Geometry check sheet. Reference: the model listing, model coordinates, mm. A direction names the side the tool comes from. Round coordinates to 2 decimals unless told otherwise and drop trailing zeros. Write each loop counter-clockwise with the first axis right and the second up, starting at its lowest first coordinate (ties: lowest second). Pieces come first, ordered by that corner, then holes. Notation, with made-up numbers: M 3,74.5 L 40,74.5 A22 cw 40,96.5 Z; hole C -3.75,-22 d1. An arc over 180 degrees is marked long. One line per item, written item: value. Start each with the question number.
1. Depth check by flat-ended pin: P1, Ø8.5, axis at x = 0.5, z = 1, coming from the -Y side; P2, Ø3, axis at x = 0, z = 0, coming from the +Y side; P3, Ø3.5, axis at x = -14, y = 20, coming from the +Z side; P4, Ø1, axis at x = -11.5, z = 4.5, coming from the -Y side. Enter the tip coordinate at first touch or a pass-through.
2. Section check B-B (x = 0). Record the boundary of the cut face in (y, z).
3. Section check D-D (z = -19). Record the boundary of the cut face in (x, y).
4. Scan lines: probe 1 along X at (y, z) = (11.5, 0); probe 2 along Y at (x, z) = (-14, 3); probe 3 along Y at (x, z) = (-5, -3.5). Record each from-to range of solid material in increasing order. Write a range as [from, to].
5. Access from +Z, -Z, +X, -X, +Y, -Y to the whole of each face (thin tool, end or side, straight path). Record for faces 1 (the cylindrical face through (19.16, 65.06, -25.94)), 2 (the cylindrical face through (2.54, 9.92, 8.06)), 3 (the flat face through (-13, 22, 9.5)).
from build123d import *

# Parameters (mm, degrees)
SKETCH_1_R           = 5.95
EXTRUDE_1_DEPTH      = 4.5
SKETCH_4_R           = 8.45
EXTRUDE_4_DEPTH      = 17.75
EXTRUDE_6_DEPTH      = 5.75
EXTRUDE_6_DEPTH_BACK = 5.75
SKETCH_12_R          = 9.5
EXTRUDE_10_DEPTH     = 1
SKETCH_7_R           = 2.3
CUT_EXTRUDE_1_DEPTH  = 57.22806055
SKETCH_8_R           = 6.5
CUT_EXTRUDE_2_DEPTH  = 6
SKETCH_9_R           = 9.5
EXTRUDE_7_DEPTH      = 36
SKETCH_10_R          = 8.45
EXTRUDE_8_DEPTH      = 40
EXTRUDE_START        = 1
SKETCH_13_R          = 9.5
SKETCH_13_R_2        = 2.3
EXTRUDE_11_DEPTH     = 1
SKETCH_14_R          = 3.25
CUT_EXTRUDE_3_DEPTH  = 8
CUT_EXTRUDE_START    = -18
CUT_EXTRUDE_4_DEPTH  = 18
CUT_EXTRUDE_START_2  = 11
SKETCH_16_R          = 14.956390748
SKETCH_16_R_2        = 7.5
CUT_EXTRUDE_5_DEPTH  = 22
FILLET_2_R           = 5
SKETCH_18_R          = 7.5
EXTRUDE_12_DEPTH     = 11.5


with BuildPart() as part:
    # Эскиз1 → Бобышка-Вытянуть1 (new body)
    with BuildSketch(Plane(origin=(0, 0, 0), x_dir=(1, 0, 0), z_dir=(0, 1, 0))):
        with Locations(Location((0, 0, 0), (0, 0, 270))):
            Circle(SKETCH_1_R)
    extrude(amount=EXTRUDE_1_DEPTH)

    # Эскиз4 → Бобышка-Вытянуть4 (add)
    with BuildSketch(Plane(origin=(0, 4.5, 0), x_dir=(1, 0, 0), z_dir=(0, 1, 0))):
        with Locations(Location((0, 0, 0), (0, 0, 270))):
            Circle(SKETCH_4_R)
    extrude(amount=EXTRUDE_4_DEPTH)

    # Эскиз6 → Бобышка-Вытянуть6 (add, two sides: drawn at the far end of the back side and taken through both)
    with BuildSketch(Plane(origin=(0, 22.25, 0), x_dir=(1, 0, 0), z_dir=(0, 1, 0)).offset(-EXTRUDE_6_DEPTH_BACK)):
        with BuildLine():
            Line((-7.002075382, 9.5), (-30, 9.5))
            Line((-30, 9.5), (-30, -9.5))
            Line((-30, -9.5), (0, -9.5))
            Line((0, -9.5), (0.833655922, -9.5))
            ThreePointArc((0.833655922, -9.5), (3.331132848, -9.18310947), (5.670324417, -8.252521801))
            ThreePointArc((5.670324417, -8.252521801), (13.556905273, -2.05094269), (19.066851837, 6.333461279))
            Line((19.066851837, 6.333461279), (28.114764095, 31.1923959))
            Line((28.114764095, 31.1923959), (10.2606043, 37.690778624))
            Line((10.2606043, 37.690778624), (2.394850826, 16.079798567))
            ThreePointArc((2.394850826, 16.079798567), (-1.266311019, 11.308479557), (-7.002075382, 9.5))
        make_face()
    extrude(amount=EXTRUDE_6_DEPTH + EXTRUDE_6_DEPTH_BACK)

    # Эскиз12 → Бобышка-Вытянуть10 (add)
    with BuildSketch(Plane(origin=(0, 28, 0), x_dir=(1, 0, 0), z_dir=(0, 1, 0))):
        with Locations(Location((15.938492836, 25.514507365, 0), (0, 0, 70))):
            Circle(SKETCH_12_R)
    extrude(amount=EXTRUDE_10_DEPTH)

    # Эскиз7 → Вырез-Вытянуть1 (cut, through all)
    with BuildSketch(Plane.XZ):
        with Locations(Location((0, 0, 0), (0, 0, 270))):
            Circle(SKETCH_7_R)
    extrude(amount=-CUT_EXTRUDE_1_DEPTH, mode=Mode.SUBTRACT)

    # Эскиз8 → Вырез-Вытянуть2 (cut)
    with BuildSketch(Plane(origin=(0, 28, 0), x_dir=(1, 0, 0), z_dir=(0, 1, 0))):
        with Locations(Location((0, 0, 0), (0, 0, 270))):
            Circle(SKETCH_8_R)
    extrude(amount=-CUT_EXTRUDE_2_DEPTH, mode=Mode.SUBTRACT)

    # Эскиз9 → Бобышка-Вытянуть7 (add)
    with BuildSketch(Plane.XZ.offset(-28)):
        with Locations(Location((-20.5, 0, 0), (0, 0, 90))):
            Circle(SKETCH_9_R)
    extrude(amount=-EXTRUDE_7_DEPTH)

    # Эскиз10 → Бобышка-Вытянуть8 (add)
    with BuildSketch(Plane(origin=(0, 29, 0), x_dir=(1, 0, 0), z_dir=(0, 1, 0))):
        with Locations(Location((15.938492836, 25.514507365, 0), (0, 0, 270))):
            Circle(SKETCH_10_R)
    extrude(amount=EXTRUDE_8_DEPTH)

    # Эскиз13 → Бобышка-Вытянуть11 (add)
    with BuildSketch(Plane.XZ.offset(-16.5).offset(EXTRUDE_START)):
        with Locations(Location((0, 0, 0), (0, 0, 90))):
            Circle(SKETCH_13_R)
        with Locations(Location((0, 0, 0), (0, 0, 270))):
            Circle(SKETCH_13_R_2, mode=Mode.SUBTRACT)
    extrude(amount=-EXTRUDE_11_DEPTH)

    # Эскиз14 → Вырез-Вытянуть3 (cut)
    with BuildSketch(Plane(origin=(0, 69, 0), x_dir=(1, 0, 0), z_dir=(0, 1, 0))):
        with Locations(Location((15.938492836, 25.514507365, 0), (0, 0, 270))):
            Circle(SKETCH_14_R)
    extrude(amount=-CUT_EXTRUDE_3_DEPTH, mode=Mode.SUBTRACT)

    # Эскиз15 → Вырез-Вытянуть4 (cut)
    with BuildSketch(Plane(origin=(0, 28, 0), x_dir=(1, 0, 0), z_dir=(0, 1, 0)).offset(CUT_EXTRUDE_START)):
        with BuildLine():
            Line((-20.5, 9.5), (-20.5, 16.947416375))
            Line((-20.5, 16.947416375), (-42.12929037, 16.947416375))
            Line((-42.12929037, 16.947416375), (-42.12929037, -12.742276146))
            Line((-42.12929037, -12.742276146), (-20.5, -12.742276146))
            Line((-20.5, -12.742276146), (-20.5, -9.5))
            ThreePointArc((-20.5, -9.5), (-30, 0), (-20.5, 9.5))
        make_face()
        with BuildLine():
            Line((7.155380289, 29.134857346), (-1.255186481, 32.601646037))
            Line((-1.255186481, 32.601646037), (4.631093303, 46.881994095))
            Line((4.631093303, 46.881994095), (38.784745505, 32.804049238))
            Line((38.784745505, 32.804049238), (32.89846572, 18.523701179))
            Line((32.89846572, 18.523701179), (24.721605383, 21.894157383))
            ThreePointArc((24.721605383, 21.894157383), (19.558842817, 34.297619911), (7.155380289, 29.134857346))
        make_face()
    extrude(amount=CUT_EXTRUDE_4_DEPTH, mode=Mode.SUBTRACT)

    # Эскиз16 → Вырез-Вытянуть5 (cut)
    with BuildSketch(Plane(origin=(0, 28, 0), x_dir=(1, 0, 0), z_dir=(0, 1, 0)).offset(CUT_EXTRUDE_START_2)):
        with Locations((-20.5, 0)):
            Circle(SKETCH_16_R)
        with Locations(Location((-20.5, 0, 0), (0, 0, 270))):
            Circle(SKETCH_16_R_2, mode=Mode.SUBTRACT)
    extrude(amount=CUT_EXTRUDE_5_DEPTH, mode=Mode.SUBTRACT)

    # Скругление2
    # the kernel refuses this fillet: 5 mm, written as the material it adds along each edge
    with BuildSketch(Plane(origin=(-20.5, 39, 0), x_dir=(0, 0, 1), z_dir=(-1, 0, 0))) as fillet_2_piece_1:
        with BuildLine():
            CenterArc((12.5, 4), FILLET_2_R, 180, 53.130102354)
            Line((7.5, 4), (7.4, 4))
            Line((7.4, 4), (7.4, 0))
            Line((7.4, 0), (7.5, -0.1))
            ThreePointArc((7.5, -0.1), (8.5, -0.1), (9.44, -0.08))
            Line((9.44, -0.08), (9.5, 0))
        make_face()
    revolve(axis=Axis((-20.5, 39, 0), (0, 1, 0)))
    with BuildSketch(Plane(origin=(-20.5, 61, 0), x_dir=(0, 0, 1), z_dir=(-1, 0, 0))) as fillet_2_piece_2:
        with BuildLine():
            CenterArc((12.5, -4), FILLET_2_R, 126.869897646, 53.130102354)
            Line((9.5, 0), (9.44, 0.08))
            ThreePointArc((9.44, 0.08), (8.5, 0.1), (7.5, 0.1))
            Line((7.5, 0.1), (7.4, 0))
            Line((7.4, 0), (7.4, -4))
            Line((7.4, -4), (7.5, -4))
        make_face()
    revolve(axis=Axis((-20.5, 61, 0), (0, 1, 0)))

    # Эскиз18 → Бобышка-Вытянуть12 (add)
    with BuildSketch(Plane.XZ.offset(-16.5)):
        with BuildLine():
            Line((9.278482036, 11.69085434), (12.972576627, 8.775389277))
            ThreePointArc((12.972576627, 8.775389277), (20.997261978, -0.921608959), (24.337711873, -13.057042378))
            Line((24.337711873, -13.057042378), (24.865572733, -22.265316003))
            Line((24.865572733, -22.265316003), (5.413533881, -23.476451416))
            Line((5.413533881, -23.476451416), (-9.371872764, -11.807465836))
            ThreePointArc((-9.371872764, -11.807465836), (-8.040562687, 6.286337643), (9.278482036, 11.69085434))
        make_face()
        Circle(SKETCH_18_R, mode=Mode.SUBTRACT)
    extrude(amount=-EXTRUDE_12_DEPTH)


solid = part.part
Result sheet:
1. P1: stops at y = 0
1. P2: passes through
1. P3: stops at z = 9.5
1. P4: stops at y = 16.5
2. outline: M 0,-5.95 L 4.5,-5.95 L 4.5,-8.45 L 15.5,-8.45 L 15.5,-9.5 L 16.5,-9.5 L 16.5,-19.2 L 28,-19.2 L 28,-6.5 L 22,-6.5 L 22,-2.3 L 0,-2.3 Z; M 0,2.3 L 22,2.3 L 22,6.5 L 28,6.5 L 28,11.72 L 16.5,11.72 L 16.5,9.5 L 15.5,9.5 L 15.5,8.45 L 4.5,8.45 L 4.5,5.95 L 0,5.95 Z
3. outline: M -0.26,16.5 L 24.68,16.5 L 24.68,28 L 22.85,28 L 22.85,29 L 21.32,29 L 21.32,69 L 10.56,69 L 10.56,29 L 9.02,29 L 9.02,28 L -0.26,28 Z
4. probe 1: x = [-8.45, -2.3], [2.3, 8.45]
4. probe 2: y = [16.5, 64]
4. probe 3: y = [4.5, 22]
5. face 1: +Y
5. face 2: -Y
5. face 3: +Z, -X, +Y, -Y
